Check sheet for the modelled part. Datum: model origin and axes. Units: mm. A direction names the side the tool comes from. Round coordinates to 2 decimals unless told otherwise and drop trailing zeros. Loops run counter-clockwise (first coordinate to the right, second up) from the corner with the lowest first, then second, coordinate; pieces in that order, holes last. Notation, with made-up numbers: (-31.75, 9.5) - (18.25, 9.5) arc R16 ccw to (18.25, 25.5) - close; hole circle Ø3 at (-29, 11). An arc over 180 degrees is marked (long way). Put each result on its own line as item: value.
```python
from build123d import *

# Parameters (mm, degrees)
BOSS_EXTRUDE1_DEPTH = 20
SKETCH2_R           = 60
BOSS_EXTRUDE2_DEPTH = 50
SKETCH3_R           = 40
BOSS_EXTRUDE3_DEPTH = 20
SKETCH4_R           = 50
SKETCH4_R_2         = 25
CUT_EXTRUDE1_DEPTH  = 70


with BuildPart() as part:
    # Sketch1 → Boss-Extrude1 (new body)
    with BuildSketch(Plane(origin=(0, 0, 0), x_dir=(1, 0, 0), z_dir=(0, 1, 0))):
        with BuildLine():
            ThreePointArc((-47.892857143, -57.717191847), (0, -75), (47.892857143, -57.717191847))
            ThreePointArc((47.892857143, -57.717191847), (91.104177178, -36.827906099), (139.071428571, -38.478127898))
            ThreePointArc((139.071428571, -38.478127898), (190, 0), (139.071428571, 38.478127898))
            ThreePointArc((139.071428571, 38.478127898), (91.104177178, 36.827906099), (47.892857143, 57.717191847))
            ThreePointArc((47.892857143, 57.717191847), (0, 75), (-47.892857143, 57.717191847))
            ThreePointArc((-47.892857143, 57.717191847), (-91.104177178, 36.827906099), (-139.071428571, 38.478127898))
            ThreePointArc((-139.071428571, 38.478127898), (-190, 0), (-139.071428571, -38.478127898))
            ThreePointArc((-139.071428571, -38.478127898), (-91.104177178, -36.827906099), (-47.892857143, -57.717191847))
        make_face()
    extrude(amount=BOSS_EXTRUDE1_DEPTH)

    # Sketch2 → Boss-Extrude2 (add)
    with BuildSketch(Plane(origin=(0, 20, 0), x_dir=(1, 0, 0), z_dir=(0, 1, 0))):
        with Locations(Location((0, 0, 0), (0, 0, 90))):
            Circle(SKETCH2_R)
    extrude(amount=BOSS_EXTRUDE2_DEPTH)

    # Sketch3 → Boss-Extrude3 (add)
    with BuildSketch(Plane(origin=(0, 20, 0), x_dir=(1, 0, 0), z_dir=(0, 1, 0))):
        with Locations(Location((-150, 0, 0), (0, 0, 74.144374523))):
            Circle(SKETCH3_R)
        with Locations(Location((150, 0, 0), (0, 0, 105.855625477))):
            Circle(SKETCH3_R)
    extrude(amount=BOSS_EXTRUDE3_DEPTH)

    # Sketch4 → Cut-Extrude1 (cut)
    with BuildSketch(Plane(origin=(0, 70, 0), x_dir=(1, 0, 0), z_dir=(0, 1, 0))):
        with Locations(Location((0, 0, 0), (0, 0, 270))):
            Circle(SKETCH4_R)
        with Locations(Location((-150, 0, 0), (0, 0, 270))):
            Circle(SKETCH4_R_2)
        with Locations(Location((150, 0, 0), (0, 0, 270))):
            Circle(SKETCH4_R_2)
    extrude(amount=-CUT_EXTRUDE1_DEPTH, mode=Mode.SUBTRACT)


solid = part.part
```
Item 1: Section check A-A on z = 0. Enter the section's corners in (x, y), then the cut area to 3 significant figures.
Filled sheet:
outline: (-190, 0) - (-175, 0) - (-175, 40) - (-190, 40) - close; (-125, 0) - (-50, 0) - (-50, 70) - (-60, 70) - (-60, 20) - (-110, 20) - (-110, 40) - (-125, 40) - close; (50, 0) - (125, 0) - (125, 40) - (110, 40) - (110, 20) - (60, 20) - (60, 70) - (50, 70) - close; (175, 0) - (190, 0) - (190, 40) - (175, 40) - close
area: 5,800 mm²
Item 2: Section check B-B on x = -150. Enter the section's corners in (y, z).
Filled sheet:
outline: (0, -40) - (40, -40) - (40, -25) - (0, -25) - close; (0, 25) - (40, 25) - (40, 40) - (0, 40) - close
Item 3: Tool access check on faces 4 (the flat face through (-138.447, 40, 22.344)), 5 (the flat face through (-33, 20, -51)), 6 (the flat face through (127.656, 40, -11.553)), 7 (the cylindrical face through (-90.44, 9.86, -36.97)), 8 (the cylindrical face through (-0.727, 9.86, 74.996)). Record the directions out of +Z, -Z, +X, -X, +Y, -Y that give a thin tool (end or side, any length) a straight path to the whole face; none if there is none.
Filled sheet:
face 4: +Z, -Z, -X, +Y
face 5: +Y
face 6: +Z, -Z, +X, +Y
face 7: -Z, +Y, -Y
face 8: +Z, +Y, -Y
Item 4: Thickness scan on line 1 (X direction, y = 31, z = 0); line 2 (X direction, y = 32, z = 35.5); line 3 (X direction, y = 15, z = -9). Record the ranges inside material, lowest first. Write a range as from..to.
Filled sheet:
line 1: -190..-175, -125..-110, -60..-50, 50..60, 110..125, 175..190
line 2: -168.43..-131.57, -48.37..-35.21, 35.21..48.37, 131.57..168.43
line 3: -188.97..-173.32, -126.68..-49.18, 49.18..126.68, 173.32..188.97
Item 5: Section check D-D on y = 13.5. Enter the section's corners in (x, z), then the cut area to 3 significant figures.
Filled sheet:
outline: (-139.07, -38.48) arc R100 cw to (-47.89, -57.72) arc R75 ccw to (47.89, -57.72) arc R100 cw to (139.07, -38.48) arc R40 ccw (long way) to (139.07, 38.48) arc R100 cw to (47.89, 57.72) arc R75 ccw to (-47.89, 57.72) arc R100 cw to (-139.07, 38.48) arc R40 ccw (long way) to start; hole circle Ø50 at (-150, 0); hole circle Ø100 at (0, 0); hole circle Ø50 at (150, 0)
area: 22,900 mm²
Item 6: Go/stop test with flat-tipped pins: pin 1 (4 mm diameter, centred on x = -58, y = 8.5, fed in from -Z); pin 2 (2 mm diameter, centred on x = 36.5, y = 47, fed in from +Z); pin 3 (6 mm diameter, centred on x = 82, y = 15, fed in from -Z); pin 4 (1 mm diameter, centred on x = -45.5, z = 39, fed in from -Y). Record where each tip stops, or that it passes through.
Filled sheet:
pin 1: z = -51.66
pin 2: z = 48.37
pin 3: z = -40.19
pin 4: y = 0
Item 7: Section check C-C on y = 32. Enter the section's corners in (x, z), then the cut area to 3 significant figures.
Filled sheet:
outline: circle Ø80 at (-150, 0); circle Ø120 at (0, 0); circle Ø80 at (150, 0); hole circle Ø50 at (-150, 0); hole circle Ø100 at (0, 0); hole circle Ø50 at (150, 0)
area: 9,580 mm²
Item 8: Release check for a two-part mould opening along X. For faces 1 (the cylindrical face through (174.787, 20.28, -3.255)), 2 (the flat face through (-45, 70, 23)), 3 (the cylindrical face through (0.727, 9.86, -74.996)) record: +X half, -X half, draft (parallel to the pull), parting line (faces both ways), or undercut.
Filled sheet:
face 1: undercut
face 2: draft
face 3: parting line
